Read the model definition and answer for the solid it produces. Units are mm, in the model's axes. A direction names the side the tool comes from. Give positions to 0.01 mm unless a question says otherwise; leave off trailing zeros. Loops run counter-clockwise (first coordinate to the right, second up) from the corner with the lowest first, then second, coordinate; pieces in that order, holes last. Notation, with made-up numbers: (-28.75, 44) -> (22.25, 44) arc R20 cw to (22.25, 55) -> close; hole circle Ø9 at (-18, 62.25). An arc over 180 degrees is marked (long way). Answer as CSV lines item,"result". Start each with the question number.
```python
from build123d import *

# Parameters (mm, degrees)
F0_R     = 6.35
F1_DEPTH = 6.35
F2_R     = 3.175
F3_DEPTH = 19.05
F4_R     = 6.35
F5_DEPTH = 25.4
F6_SIZE2 = 1.1196763275
F6_SIZE  = 6.35


with BuildPart() as f1:
    # F0 (on Top) → F1 (new body)
    with BuildSketch(Plane.XY):
        Circle(F0_R)
    extrude(amount=F1_DEPTH)

    # F2 (on face) → F3 (join)
    with BuildSketch(Plane.XY.offset(6.35)):
        Circle(F2_R)
    extrude(amount=F3_DEPTH)

    # F4 (on face) → F5 (join)
    with BuildSketch(Plane.XY.offset(25.4)):
        Circle(F4_R)
    extrude(amount=F5_DEPTH)

    # F6
    f6_edges = [f1.edges().sort_by_distance(p)[0] for p in [
        (-6.35, 0, 0),
    ]]
    f6_side = f1.faces().sort_by_distance((0, 0, 0))[0]
    chamfer(f6_edges, length=F6_SIZE, length2=F6_SIZE2, reference=f6_side)


solid = f1.part
```
(1) A tool of negligible diameter and unlimited length cuts with its end or side. For faces 4 (the face through (-1.38, -6.2, 3.7)), 5 (the face through (-0.69, -3.1, 15.74)), from which of +Z, -Z, +X, -X, +Y, -Y can it reach the whole face along a straight path? Write none if from no direction.
(2) Find section B-B on z = 43.5. Write down the section's boundary in (x, y), then the cut area to 3 significant figures.
(3) The mould has two halves that part along Z. Classify faces 1 (the face through (0, 0, 50.8)), 2 (the face through (-1.38, -6.2, 37.92)), 3 (the face through (-2, 3, 25.4)): pulls with the +Z half, pulls with the -Z half, needs draft (parallel to the pull), parting line crosses it, or undercut.
(4) Each of these flat-tipped pins is pushed along its axis until it touches: P1, Ø1.5, axis at x = 1.5, y = 5, coming from the -Z side; P2, Ø3, axis at x = -2, z = 8.5, coming from the -Y side; P3, Ø1.5, axis at x = -1, y = 0, coming from the -Z side. Where does it stop, or does it pass through?
(5) Find the intervals of material crossed by line 1 along Z through (x, y) = (0.25, -5); line 2 along Z through (x, y) = (6.25, 0); line 3 along Y through (x, z) = (2.25, 19), in increasing order. Write a range as from..to.
(6) Find section A-A on z = 18. Write down the section's boundary in (x, y) (3 decimals), then the cut area to 3 significant figures.
Answer block:
1,face 4,"+Z, -Z"
1,face 5,"none"
2,outline,"circle Ø12.7 at (0, 0)"
2,area,"127 mm2"
3,face 1,"pulls with the +Z half"
3,face 2,"needs draft"
3,face 3,"undercut"
4,P1,"stops at z = 0.79"
4,P2,"stops at y = -3.14"
4,P3,"stops at z = 0.04"
5,line 1,"z = 0.88..6.35, 25.4..50.8"
5,line 2,"z = 1.1..6.35, 25.4..50.8"
5,line 3,"y = -2.24..2.24"
6,outline,"circle Ø6.35 at (0, 0)"
6,area,"31.7 mm2"
